Geometry: final body of the model. Coordinates: model frame, mm. A direction names the side the tool comes from. Round coordinates to 2 decimals unless told otherwise and drop trailing zeros. Write each loop counter-clockwise with the first axis right and the second up, starting at its lowest first coordinate (ties: lowest second). Pieces come first, ordered by that corner, then holes. Notation, with made-up numbers: (38.5, 43.25) -> (63.5, 43.25) arc R23 ccw to (63.5, 76.25) -> close; hole circle Ø2 at (-18.75, 0.25). An arc over 180 degrees is marked (long way). One line per item, written item: value. Start each with the question number.
from build123d import *

# Parameters (mm, degrees)
SKETCH1_R           = 42.9384162
BOSS_EXTRUDE1_DEPTH = 12.7
SKETCH6_W           = 6.747965948
SKETCH6_H           = 12.700002404
BOSS_EXTRUDE2_DEPTH = 3.81
CIRPATTERN8_COUNT   = 4
CUT_EXTRUDE3_START  = -24
CUT_EXTRUDE3_DEPTH  = 24
SKETCH10_R          = 40.386
CUT_EXTRUDE4_DEPTH  = 38.1


with BuildPart() as part:
    # Sketch1 → Boss-Extrude1 (new body)
    with BuildSketch(Plane(origin=(0, 0, 0), x_dir=(1, 0, 0), z_dir=(0, 1, 0))):
        with Locations(Location((0, 0, 0), (0, 0, 270))):
            Circle(SKETCH1_R)
    extrude(amount=BOSS_EXTRUDE1_DEPTH)

    # Sketch6 → Boss-Extrude2 (add, symmetric)
    with BuildSketch(Plane.XY):
        with Locations((45.914433226, 6.349998798)):
            Rectangle(SKETCH6_W, SKETCH6_H)
    boss_extrude2 = extrude(amount=BOSS_EXTRUDE2_DEPTH, both=True)

    # CirPattern8: Boss-Extrude2 ×4 about axis
    cirpattern8_axis = Axis((0, 0, 0), (0, 1, 0))
    for i in range(1, CIRPATTERN8_COUNT):
        add(boss_extrude2.rotate(cirpattern8_axis, i * 360 / CIRPATTERN8_COUNT))

    # Sketch8 → Cut-Extrude3 (cut)
    with BuildSketch(Plane(origin=(0, 12.7, 0), x_dir=(1, 0, 0), z_dir=(0, 1, 0)).offset(CUT_EXTRUDE3_START)):
        with BuildLine():
            Line((-41.736458882, -3.81), (-42.769048222, -3.81))
            ThreePointArc((-42.769048222, -3.81), (-30.362045269, -30.362045269), (-3.81, -42.769048222))
            Line((-3.81, -42.769048222), (-3.81, -41.736458882))
            ThreePointArc((-3.81, -41.736458882), (-29.6348452, -29.6348452), (-41.736458882, -3.81))
        make_face()
        with BuildLine():
            Line((3.81, -41.736458882), (3.81, -42.769048222))
            ThreePointArc((3.81, -42.769048222), (30.362045269, -30.362045269), (42.769048222, -3.81))
            Line((42.769048222, -3.81), (41.736458882, -3.81))
            ThreePointArc((41.736458882, -3.81), (29.6348452, -29.6348452), (3.81, -41.736458882))
        make_face()
        with BuildLine():
            ThreePointArc((42.769048222, 3.81), (30.362045269, 30.362045269), (3.81, 42.769048222))
            Line((3.81, 42.769048222), (3.81, 41.736458882))
            ThreePointArc((3.81, 41.736458882), (29.6348452, 29.6348452), (41.736458882, 3.81))
            Line((41.736458882, 3.81), (42.769048222, 3.81))
        make_face()
        with BuildLine():
            ThreePointArc((-3.81, 42.769048222), (-30.362045269, 30.362045269), (-42.769048222, 3.81))
            Line((-42.769048222, 3.81), (-41.736458882, 3.81))
            ThreePointArc((-41.736458882, 3.81), (-29.6348452, 29.6348452), (-3.81, 41.736458882))
            Line((-3.81, 41.736458882), (-3.81, 42.769048222))
        make_face()
    extrude(amount=CUT_EXTRUDE3_DEPTH, mode=Mode.SUBTRACT)

    # Sketch10 → Cut-Extrude4 (cut)
    with BuildSketch(Plane(origin=(0, 12.7, 0), x_dir=(1, 0, 0), z_dir=(0, 1, 0))):
        with Locations(Location((0, 0, 0), (0, 0, 270))):
            Circle(SKETCH10_R)
    extrude(amount=-CUT_EXTRUDE4_DEPTH, mode=Mode.SUBTRACT)


solid = part.part
(1) Section query D-D (x = -20). Output: boundary loops of the cut face in (y, z), and give its area (3 significant figures).
(2) Pin query (flat end, axial travel): pin 1 (5 mm diameter, centred on x = 15.5, y = 8, fed in from +Z); pin 2 (5 mm diameter, centred on y = 5.5, z = 39, fed in from +X); pin 3 (2.5 mm diameter, centred on y = 5.5, z = -45.5, fed in from +X); pin 4 (1 mm diameter, centred on x = -9.5, z = -38.5, fed in from +Y). Return the tip coordinate at first contact, or that it passes through.
(3) Section query C-C (y = 6.75). Output: boundary loops of the cut face in (x, z), and give its area (3 significant figures).
(4) Set-up query: faces 1 (the face through (0, 0, 46)), 2 (the face through (45, 6, -3.81)), 3 (the face through (-3.81, 6, 45)), 4 (the face through (3.81, 6, 45)), 5 (the face through (-46, 6, -3.81)). Return all of +Z, -Z, +X, -X, +Y, -Y with unobstructed straight access to the full face (end or side cutting, diameter ignored); none if empty.
(5) Line query: probe 1 along X at (y, z) = (2.5, 0); probe 2 along Z at (x, y) = (-27, 2.25); probe 3 along Z at (x, y) = (32.5, 5.25). Output: solid intervals per line, ascending.
Results list:
1. outline: (0, -36.83) -> (12.7, -36.83) -> (12.7, -35.09) -> (0, -35.09) -> close; (0, 35.09) -> (12.7, 35.09) -> (12.7, 36.83) -> (0, 36.83) -> close
1. area: 44.3 mm^2
2. pin 1: stops at z = 39.84
2. pin 2: stops at x = 20.6
2. pin 3: stops at x = 3.81
2. pin 4: passes through
3. outline: (-49.29, -3.81) -> (-41.74, -3.81) arc R41.91 ccw to (-3.81, -41.74) -> (-3.81, -49.29) -> (3.81, -49.29) -> (3.81, -41.74) arc R41.91 ccw to (41.74, -3.81) -> (49.29, -3.81) -> (49.29, 3.81) -> (41.74, 3.81) arc R41.91 ccw to (3.81, 41.74) -> (3.81, 49.29) -> (-3.81, 49.29) -> (-3.81, 41.74) arc R41.91 ccw to (-41.74, 3.81) -> (-49.29, 3.81) -> close; hole circle Ø80.77 at (0, 0)
3. area: 621 mm^2
4. face 1: +Z, -Z, +X, -X, -Y
4. face 2: -Z, +X, +Y, -Y
4. face 3: +Z, -X, +Y, -Y
4. face 4: +Z, +X, +Y, -Y
4. face 5: -Z, -X, +Y, -Y
5. probe 1: x = -49.29 to -40.39, 40.39 to 49.29
5. probe 2: z = -32.05 to -30.03, 30.03 to 32.05
5. probe 3: z = -26.46 to -23.97, 23.97 to 26.46
